Here's how the part is built. I have some questions about the finished solid (model axes, mm). Face numbers are marked on the shaded views. Give positions to 0.01 mm unless a question says otherwise; leave off trailing zeros. Write each loop counter-clockwise with the first axis right and the second up, starting at its lowest first coordinate (ties: lowest second). Pieces come first, ordered by that corner, then holes. Notation, with made-up numbers: (40, -14.5) -> (90, -14.5) arc R34 cw to (90, 23.5) -> close; hole circle Ø3 at (30, 20). An arc over 180 degrees is marked (long way). Use CSV: the item, a comma, the result in double quotes. Start each with the question number.
(1) For pin 1 Ø4 at (x, y) = (3, -6) entering from -Z, with a flat end and sliding along its axis, tell me the tip position at first contact or that it passes through.
(2) Suppose I cut it at C-C on x = -5.25. List the corners of the cut face in (y, z) for me, plus the area to 3 significant figures.
(3) Suppose I cut it at A-A on y = -8.25. List the corners of the cut face in (x, z) for me.
(4) Suppose I cut it at B-B on z = 1.7. List the corners of the cut face in (x, y) for me, plus the area to 3 significant figures.
(5) If we mould it in two halves opening along Z, with no side actions, what happens to the marked faces 1, 2 and 3? For each: pulls with the +Z half, pulls with the -Z half, needs draft (parallel to the pull), parting line crosses it, or undercut.
(6) I need wall thicknesses on L1, parallel to Y at x = 8, z = 1.35. Which ranges of the line are inside material? Lowest first, please. Write a range as [from, to].
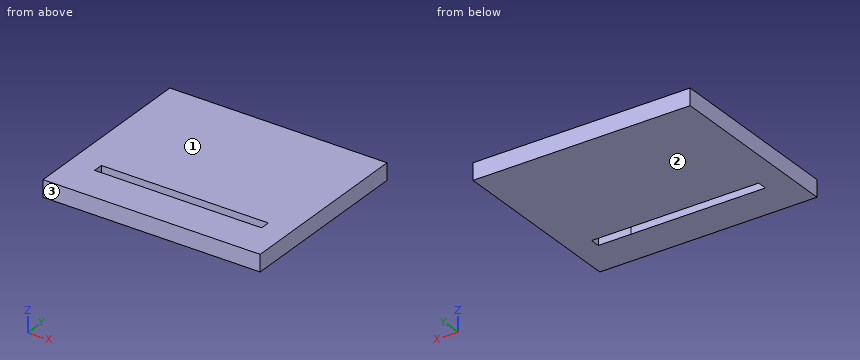
from build123d import *

# Parameters (mm, degrees)
F1_DEPTH = 2


with BuildPart() as f1:
    # F0 (on Top) → F1 (new body)
    with BuildSketch(Plane.XY):
        Polygon((13, -8.5), (13, 8.5), (-13, 8.5), (-13, -8.5), (-13, -13.5), (6.247106, -13.5), (13, -13.5), align=None)
        Polygon((10.138918, -9.100043), (6.247106, -9.1), (-9.861082, -9.099823), (-9.861082, -7.931823), (10.138918, -7.932043), align=None, mode=Mode.SUBTRACT)
    extrude(amount=F1_DEPTH)


solid = f1.part
Geometry says:
1,pin 1,"z = 0"
2,outline,"(-13.5, 0) -> (-9.1, 0) -> (-9.1, 2) -> (-13.5, 2) -> close; (-7.93, 0) -> (8.5, 0) -> (8.5, 2) -> (-7.93, 2) -> close"
2,area,"41.7 mm²"
3,outline,"(-13, 0) -> (-9.86, 0) -> (-9.86, 2) -> (-13, 2) -> close; (10.14, 0) -> (13, 0) -> (13, 2) -> (10.14, 2) -> close"
4,outline,"(-13, -13.5) -> (13, -13.5) -> (13, 8.5) -> (-13, 8.5) -> close; hole (-9.86, -9.1) -> (10.14, -9.1) -> (10.14, -7.93) -> (-9.86, -7.93) -> close"
4,area,"549 mm²"
5,face 1,"pulls with the +Z half"
5,face 2,"pulls with the -Z half"
5,face 3,"needs draft"
6,L1,"[-13.5, -9.1], [-7.93, 8.5]"
